Can you work these out from the model? Positions are in its coordinate system, mm. Face numbers are marked on the shaded views. A direction names the side the tool comes from. Round coordinates to 2 decimals unless told otherwise and drop trailing zeros. Order: outer loops, then holes, each group sorted by start corner. A loop starts at its lowest first (then second) coordinate and runs counter-clockwise, first axis right, second up. Notation, with made-up numbers: (44.5, 15) -> (68.5, 15) arc R28 cw to (68.5, 36) -> close; hole circle Ø1 at (59.5, 60). An arc over 180 degrees is marked (long way). Use a Markdown table: item, result. Add a question column.
Q1. For the marked faces 1 and 2, which set-ups out of +Z, -Z, +X, -X, +Y, -Y let a thin tool reach every point of the face, with its end or its side?
Q2. I need wall thicknesses on line 1 along X through (y, z) = (0, 15.5); line 2 along Z through (x, y) = (0, 13.55); line 3 along X through (y, z) = (0.5, 74). Which ranges of each line are inside material? Lowest first, please. Write a range as [from, to].
Q3. We'd pull the mould along Y, two halves only. Please class the marked faces 3, 4 and 5: +Y half, -Y half, draft (parallel to the pull), parting line (faces both ways), or undercut.
Q4. If we section it at A-A on y = 0: List the corners of the cut face in (x, z) for me.
Q5. If we section it at B-B on z = 79: List the corners of the cut face in (x, y) for me.
Q6. I'm going to push flat-ended pins straight in: pin 1 Ø4 at (x, z) = (-7.5, 99) entering from -Y; pin 2 Ø4 at (x, z) = (0, 24.42) entering from -Y; pin 3 Ø8 at (y, z) = (-7, 74.5) entering from -X; pin 4 Ø5.5 at (x, z) = (-6.5, -2) entering from -Y. Where does each tip first touch, or does it pass through?
```python
from build123d import *

# Parameters (mm, degrees)
F2_ANGLE = 180
F3_DEPTH = 2.5
F4_R     = 2.616774
F5_DEPTH = 25
F6_R     = 2.5
F7_DEPTH = 25


with BuildPart() as f1:
    # F0 (on Front) → F1 (revolve)
    with BuildSketch(Plane.XZ):
        Polygon((0, 1), (0, 0), (13, 0), (13, 20), (14.25, 20.5), (14.25, 116.5), (13.25, 116.5), (13.25, 21.5), (12, 21), (12, 1), align=None)
    revolve(axis=Axis((0, 0, 0.5), (0, 0, -1)))

    # F0 (on Front) → F2 (revolve, symmetric)
    with BuildSketch(Plane.XZ) as f2_sk:
        Polygon((13, 0), (0, 0), (0, -5), (9.214125, -5), align=None)
    revolve(axis=Axis((0, 0, -2.5), (0, 0, 1)), revolution_arc=F2_ANGLE / 2)
    revolve(f2_sk.sketch, axis=Axis((0, 0, -2.5), (0, 0, -1)), revolution_arc=F2_ANGLE / 2)

    # F0 (on Front) → F3 (join, symmetric)
    with BuildSketch(Plane.XZ):
        Polygon((0, -5), (0, 0), (-12, 0), (-9, -5), align=None)
        Polygon((-8.43381, -4), (-10.23381, -1), (-1, -1), (-1, -4), align=None, mode=Mode.SUBTRACT)
    extrude(amount=F3_DEPTH, both=True)

    # F4 (on face) → F5 (cut)
    with BuildSketch(Plane(origin=(0, 0, 0), x_dir=(1, 0, 0), z_dir=(0, 0, -1))):
        with Locations((-5.104913, 6.11541)):
            Circle(F4_R)
    extrude(amount=-F5_DEPTH, mode=Mode.SUBTRACT)

    # F6 (on Front) → F7 (cut, symmetric)
    with BuildSketch(Plane.XZ):
        with Locations((0, 34.415651)):
            Circle(F6_R)
        with Locations((0, 24.415651)):
            Circle(F6_R)
    extrude(amount=F7_DEPTH, both=True, mode=Mode.SUBTRACT)


solid = f1.part
```
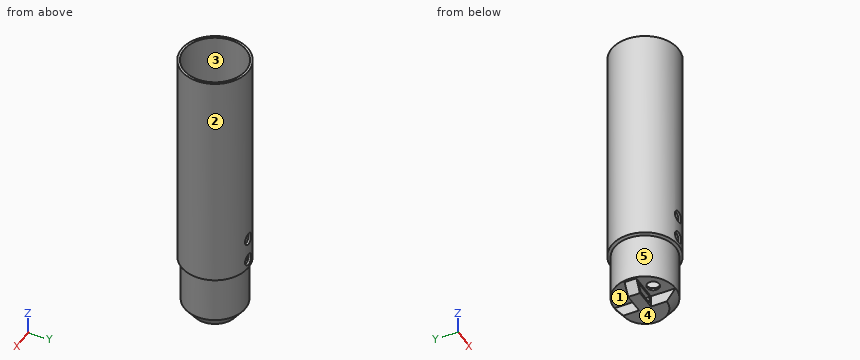
Answer below:
| question | item | result |
|---|---|---|
| 1 | face 1 | -Z, -X |
| 1 | face 2 | +Z, -Z |
| 2 | line 1 | [-13, -12], [12, 13] |
| 2 | line 2 | [20.22, 21.92], [26.92, 31.92], [36.92, 116.5] |
| 2 | line 3 | [-14.24, -13.24], [13.24, 14.24] |
| 3 | face 3 | undercut |
| 3 | face 4 | draft |
| 3 | face 5 | parting line |
| 4 | outline | (-14.25, 20.5) -> (-13, 20) -> (-13, 0) -> (-12, 0) -> (-9, -5) -> (9.21, -5) -> (13, 0) -> (13, 20) -> (14.25, 20.5) -> (14.25, 116.5) -> (13.25, 116.5) -> (13.25, 21.5) -> (12, 21) -> (12, 1) -> (-12, 1) -> (-12, 21) -> (-13.25, 21.5) -> (-13.25, 116.5) -> (-14.25, 116.5) -> close; hole (-10.23, -1) -> (-8.43, -4) -> (-1, -4) -> (-1, -1) -> close |
| 5 | outline | circle Ø28.5 at (0, 0); hole circle Ø26.5 at (0, 0) |
| 6 | pin 1 | y = -13.15 |
| 6 | pin 2 | through |
| 6 | pin 3 | x = -13.93 |
| 6 | pin 4 | y = -12.15 |
